from build123d import *

# Parameters (mm, degrees)
SKETCH1_W                     = 33.5
SKETCH1_H                     = 33.5
BOSS_EXTRUDE1_DEPTH           = 70
M3X0_5_TAPPED_HOLE1_D         = 2.5
M3X0_5_TAPPED_HOLE1_DEPTH     = 7.62
M3X0_5_TAPPED_HOLE1_TIP       = 0.751075774
M3X0_5_TAPPED_HOLE2_D         = 2.5
M3X0_5_TAPPED_HOLE2_DEPTH     = 7.62
M3X0_5_TAPPED_HOLE2_TIP       = 0.751075774
SKETCH7_W                     = 6
SKETCH7_H                     = 50
BOSS_EXTRUDE2_DEPTH           = 3
SKETCH8_W                     = 6
SKETCH8_H                     = 50
BOSS_EXTRUDE3_DEPTH           = 3
SKETCH10_W                    = 1.7
SKETCH10_H                    = 33.5
M3_CLEARANCE_HOLE1_AT_2_COUNT = 2
M3_CLEARANCE_HOLE1_AT_2_PITCH = 25
M3_CLEARANCE_HOLE1_AT_3_COUNT = 2
M3_CLEARANCE_HOLE1_AT_3_PITCH = 39.5
M3_CLEARANCE_HOLE1_AT_4_COUNT = 2
M3_CLEARANCE_HOLE1_AT_4_PITCH = 46.746657635
SKETCH11_R                    = 12.573
CUT_EXTRUDE1_DEPTH            = 71
SKETCH12_W                    = 33.5
SKETCH12_H                    = 45
CUT_EXTRUDE2_DEPTH            = 32.5
SKETCH13_W                    = 45.5
SKETCH13_H                    = 70.777616709
CUT_EXTRUDE3_DEPTH            = 34.5
SKETCH14_W                    = 45.5
SKETCH14_H                    = 5
BOSS_EXTRUDE4_DEPTH           = 2
M3_CLEARANCE_HOLE2_D          = 3.4


with BuildPart() as part:
    # Sketch1 → Boss-Extrude1 (new body)
    with BuildSketch(Plane(origin=(0, 0, 0), x_dir=(1, 0, 0), z_dir=(0, 1, 0))):
        Rectangle(SKETCH1_W, SKETCH1_H)
    extrude(amount=BOSS_EXTRUDE1_DEPTH)

    # M3x0.5 Tapped Hole1
    with Locations(Plane(origin=(13.75, 70, 13.75), x_dir=(0, 0, 1), z_dir=(0, 1, 0))):
        with Locations((0, 0), (-27.5, -27.5)):
            Hole(M3X0_5_TAPPED_HOLE1_D / 2, depth=M3X0_5_TAPPED_HOLE1_DEPTH)
            with Locations((0, 0, -(M3X0_5_TAPPED_HOLE1_DEPTH + M3X0_5_TAPPED_HOLE1_TIP / 2))):  # 118° drill point
                Cone(0, M3X0_5_TAPPED_HOLE1_D / 2, M3X0_5_TAPPED_HOLE1_TIP, mode=Mode.SUBTRACT)

    # M3x0.5 Tapped Hole2
    with Locations(Plane(origin=(16.75, 6, 13.75), x_dir=(0, 0, 1), z_dir=(1, 0, 0))):
        with Locations((0, 0), (-27.5, 0)):
            Hole(M3X0_5_TAPPED_HOLE2_D / 2, depth=M3X0_5_TAPPED_HOLE2_DEPTH)
            with Locations((0, 0, -(M3X0_5_TAPPED_HOLE2_DEPTH + M3X0_5_TAPPED_HOLE2_TIP / 2))):  # 118° drill point
                Cone(0, M3X0_5_TAPPED_HOLE2_D / 2, M3X0_5_TAPPED_HOLE2_TIP, mode=Mode.SUBTRACT)

    # Sketch11 → Cut-Extrude1 (cut, through all)
    with BuildSketch(Plane.XZ):
        Circle(SKETCH11_R)
    extrude(amount=-CUT_EXTRUDE1_DEPTH, mode=Mode.SUBTRACT)

    # Sketch12 → Cut-Extrude2 (cut)
    with BuildSketch(Plane.XY.offset(16.75)):
        with Locations((0, 35.5)):
            Rectangle(SKETCH12_W, SKETCH12_H)
    extrude(amount=-CUT_EXTRUDE2_DEPTH, mode=Mode.SUBTRACT)


with BuildPart() as body_2:
    # Sketch7 → Boss-Extrude2 (new body)
    with BuildSketch(Plane(origin=(0, 0, -16.75), x_dir=(-1, 0, 0), z_dir=(0, 0, -1))):
        with Locations((-19.75, 36)):
            Rectangle(SKETCH7_W, SKETCH7_H)
    extrude(amount=-BOSS_EXTRUDE2_DEPTH)

    # Sketch10 → M3 Clearance Hole1 (revolve, cut)
    with BuildSketch(Plane(origin=(19.75, 51, -16.75), x_dir=(0, 1, 0), z_dir=(1, 0, 0))):
        with Locations((0.85, 16.75)):
            Rectangle(SKETCH10_W, SKETCH10_H)
    m3_clearance_hole1 = revolve(axis=Axis((19.75, 51, -23.1), (0, 0, 1)), mode=Mode.SUBTRACT)

    # M3 Clearance Hole1 at 2: M3 Clearance Hole1 ×2
    with Locations(*[(0, -i * M3_CLEARANCE_HOLE1_AT_2_PITCH, 0) for i in range(1, M3_CLEARANCE_HOLE1_AT_2_COUNT)]):
        add(m3_clearance_hole1, mode=Mode.SUBTRACT)


with BuildPart() as body_3:
    # Sketch8 → Boss-Extrude3 (new body)
    with BuildSketch(Plane(origin=(0, 0, -16.75), x_dir=(-1, 0, 0), z_dir=(0, 0, -1))):
        with Locations((19.75, 36)):
            Rectangle(SKETCH8_W, SKETCH8_H)
    extrude(amount=-BOSS_EXTRUDE3_DEPTH)

    # M3 Clearance Hole1 at 3: M3 Clearance Hole1 ×2
    with Locations(*[(-i * M3_CLEARANCE_HOLE1_AT_3_PITCH, 0, 0) for i in range(1, M3_CLEARANCE_HOLE1_AT_3_COUNT)]):
        add(m3_clearance_hole1, mode=Mode.SUBTRACT)

    # M3 Clearance Hole1 at 4: M3 Clearance Hole1 ×2
    with Locations(*[Vector(-0.844980197, -0.534797593, 0) * (i * M3_CLEARANCE_HOLE1_AT_4_PITCH) for i in range(1, M3_CLEARANCE_HOLE1_AT_4_COUNT)]):
        add(m3_clearance_hole1, mode=Mode.SUBTRACT)


with BuildPart() as cut_extrude3_tool:
    # Sketch13 → Cut-Extrude3 (new body, through all)
    with BuildSketch(Plane.XY.offset(16.75)):
        with Locations((0, 29.611191645)):
            Rectangle(SKETCH13_W, SKETCH13_H)
    extrude(amount=-CUT_EXTRUDE3_DEPTH)


with BuildPart() as part_1:
    add(part.part)

    # Cut-Extrude3: cut by cut_extrude3_tool
    add(cut_extrude3_tool.part, mode=Mode.SUBTRACT)

    # Sketch14 → Boss-Extrude4 (add)
    with BuildSketch(Plane.XY.offset(16.75)):
        with Locations((0, 67.5)):
            Rectangle(SKETCH14_W, SKETCH14_H)
    extrude(amount=BOSS_EXTRUDE4_DEPTH)

    # M3 Clearance Hole2 (through all)
    with Locations(Plane(origin=(-19.75, 67.5, 16.75), x_dir=(-1, 0, 0), z_dir=(0, 0, -1))):
        with Locations((0, 0), (-39.5, 0)):
            Hole(M3_CLEARANCE_HOLE2_D / 2)


with BuildPart() as body_2_1:
    add(body_2.part)

    # Cut-Extrude3: cut by cut_extrude3_tool
    add(cut_extrude3_tool.part, mode=Mode.SUBTRACT)


with BuildPart() as body_3_1:
    add(body_3.part)

    # Cut-Extrude3: cut by cut_extrude3_tool
    add(cut_extrude3_tool.part, mode=Mode.SUBTRACT)


solid = part_1.part
Work out the finished part from the listing and answer in its coordinate system (mm). A direction names the side the tool comes from. Give positions to 0.01 mm unless a question says otherwise; leave off trailing zeros. Loops run counter-clockwise (first coordinate to the right, second up) from the corner with the lowest first, then second, coordinate; pieces in that order, holes last. Notation, with made-up numbers: (2, 18.25) - (43, 18.25) arc R18 cw to (43, 32.25) - close; hole circle Ø1 at (-19.5, -8). An arc over 180 degrees is marked (long way). Answer in a Markdown table with one row per item.
(1) Section C-C (x = 0) is taken. Give the vertices of the cut face in (y, z), and give its area (3 significant figures).
Results list:
| item | result |
|---|---|
| outline | (65, -16.75) - (70, -16.75) - (70, -12.57) - (65, -12.57) - close; (65, 12.57) - (70, 12.57) - (70, 18.75) - (65, 18.75) - close |
| area | 51.8 mm² |
(2) Flat-ended cylindrical pins translate along their axes: pin 1 Ø12 at (x, z) = (7.5, -3) entering from -Y; pin 2 Ø2.5 at (y, z) = (66.5, -6.5) entering from -X. Find the tip coordinate at first contact, or state that the pin passes through.
Results list:
| item | result |
|---|---|
| pin 1 | stops at y = 65 |
| pin 2 | stops at x = -16.75 |
(3) For a pull along X with two mould halves and no side action, classify faces 1 (the face through (18, 69, 16.75)), 2 (the face through (-16.75, 67, 0)), 3 (the face through (-18.97, 65.99, 17.76)) as pulls with the +X half, pulls with the -X half, needs draft (parallel to the pull), parting line crosses it, or undercut.
Results list:
| item | result |
|---|---|
| face 1 | needs draft |
| face 2 | pulls with the -X half |
| face 3 | undercut |
(4) A tool of negligible diameter and unlimited length cuts with its end or side. For faces 4 (the face through (-21, 69, 16.75)), 5 (the face through (16.75, 67, 0)), 6 (the face through (0, 65, 13)), from which of +Z, -Z, +X, -X, +Y, -Y can it reach the whole face along a straight path? Write none if from no direction.
Results list:
| item | result |
|---|---|
| face 4 | -Z, -X, +Y, -Y |
| face 5 | -Z, +X, +Y, -Y |
| face 6 | +Z, -Z, +X, -X, -Y |
(5) Section A-A (y = 67.5) is taken. Give the vertices of the cut face in (x, z), and give its area (3 significant figures).
Results list:
| item | result |
|---|---|
| outline | (-22.75, 16.75) - (-21.45, 16.75) - (-21.45, 18.75) - (-22.75, 18.75) - close; (-18.05, 16.75) - (-16.75, 16.75) - (-16.75, -16.75) - (16.75, -16.75) - (16.75, 16.75) - (18.05, 16.75) - (18.05, 18.75) - (-18.05, 18.75) - close; (21.45, 16.75) - (22.75, 16.75) - (22.75, 18.75) - (21.45, 18.75) - close; hole circle Ø2.5 at (-13.75, -13.75); hole circle Ø25.15 at (0, 0); hole circle Ø2.5 at (13.75, 13.75) |
| area | 693 mm² |
(6) Section B-B (z = -13.75) is taken. Give the vertices of the cut face in (x, y).
Results list:
| item | result |
|---|---|
| outline | (-16.75, 65) - (-15, 65) - (-15, 70) - (-16.75, 70) - close; (-12.5, 65) - (16.75, 65) - (16.75, 70) - (-12.5, 70) - close |
(7) Consider L1, parallel to X at y = 67.5, z = 18.2; L2, parallel to X at y = 68.25, z = -13.75; L3, parallel to Z at x = -4, y = 65.8. Determine where each line is inside the solid, lowest interval first. Write a range as [from, to].
Results list:
| item | result |
|---|---|
| L1 | x = [-22.75, -21.45], [-18.05, 18.05], [21.45, 22.75] |
| L2 | x = [-16.75, -15], [-12.5, 16.75] |
| L3 | z = [-16.75, -11.92], [11.92, 18.75] |
